Part print with two shaded views. Sizes in mm from the minimum x, y, z corner. Give positions to 0.01 mm unless a question says otherwise; leave off trailing zeros. Loops run counter-clockwise (first coordinate to the right, second up) from the corner with the lowest first, then second, coordinate; pieces in that order, holes last. Notation, with made-up numbers: (41, 35) -> (67, 35) arc R10 ccw to (67, 49) -> close; hole circle Ø9 at (50, 56.25). An arc over 180 degrees is marked (long way). One line per question, with ' | ' between items. Start each with the question number.
(1) Drill centre lines: L1, parallel to X at y = 390.5, z = 14; L2, parallel to Y at x = 583.5, z = 8. Where is each one in solid material? Low to high. Write a range as from..to.
(2) Slice it at B-B, the plane z = 23.25. Write the cut outline in (x, y), then the cut area to 3 significant figures.
(3) Slice it at A-A, the plane y = 309. Write the cut outline in (x, z), then the cut area to 3 significant figures.
(4) Flat gauge pins, fed straight in: pin 1 Ø1.5 at (x, z) = (421.5, 11.5) entering from -Y; pin 2 Ø12 at (x, z) = (152.5, 13) entering from +Y. Where does each tip first touch, or does it go through?
(5) Slice it at C-C, the plane x = 258.5. Write the cut outline in (y, z), then the cut area to 3 significant figures.
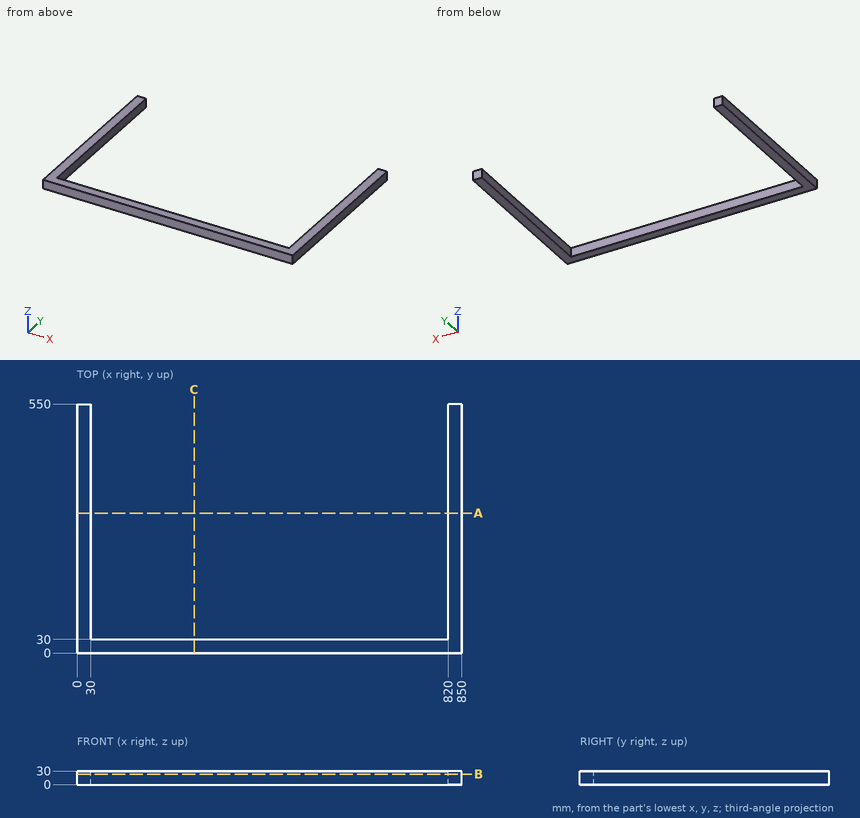
Final values:
1) L1: 0..30, 820..850 | L2: 0..30
2) outline: (0, 0) -> (850, 0) -> (850, 550) -> (820, 550) -> (820, 30) -> (30, 30) -> (30, 550) -> (0, 550) -> close | area: 56,700 mm2
3) outline: (0, 0) -> (30, 0) -> (30, 30) -> (0, 30) -> close; (820, 0) -> (850, 0) -> (850, 30) -> (820, 30) -> close | area: 1,800 mm2
4) pin 1: y = 0 | pin 2: y = 30
5) outline: (0, 0) -> (30, 0) -> (30, 30) -> (0, 30) -> close | area: 900 mm2
